Geometry: final body of the model. Coordinates: model frame, mm. A direction names the side the tool comes from. Round coordinates to 2 decimals unless told otherwise and drop trailing zeros. Write each loop counter-clockwise with the first axis right and the second up, starting at its lowest first coordinate (ties: lowest second). Pieces come first, ordered by that corner, then holes. Notation, with made-up numbers: M -5.5,85 L 44.5,85 A11 cw 44.5,105 Z; hole C 24.5,37 d5. An arc over 180 degrees is marked long. Answer as CSV lines item,"result". Start each with the question number.
Q1. Ray query, probe 1 along Y at (x, z) = (8.5, -0.5); probe 2 along Z at (x, y) = (10.25, 9); probe 3 along Y at (x, z) = (6.25, 6.5) (3 decimals). Return the intervals inside material, ascending.
Q2. Reachability of faces 1 (the flat face through (4.13, 9.44, -0.44)), 2 (the flat face through (8.1, 8.152, -0.4)), 3 (the flat face through (8, 9.309, -0.4)) from +Z, -Z, +X, -X, +Y, -Y: full face, straight path, thin tool, end or side. Return the list, or none.
Q3. Section query A-A on z = 7. Output: boundary loops of the cut face in (x, y) (3 decimals), and give its area (3 significant figures).
Q4. Section query B-B on y = 6.1. Output: boundary loops of the cut face in (x, z) (3 decimals), and give its area (3 significant figures).
Q5. First-contact query: pin 1 (1.1 mm diameter, centred on y = 7.5, z = 7.5, fed in from -X); pin 2 (1 mm diameter, centred on x = 2, z = 6, fed in from +Y); pin 3 (0.5 mm diameter, centred on x = 7, z = -0.5, fed in from -Y); pin 4 (1.1 mm diameter, centred on x = 6.5, z = 7, fed in from -Y). Flat tips, straight axial feed; report the tip coordinate or a pass-through.
Q6. Section query C-C on x = 10. Output: boundary loops of the cut face in (y, z), and give its area (3 significant figures).
Q7. Mould query, pull axis X, two halves, no side actions, for faces 4 (the flat face through (5.929, 8.4, -0.4)), 5 (the flat face through (6, 4.075, 7)), 6 (the flat face through (12.14, 6, 2)), 7 (the flat face through (4.9, 6.84, -0.4)). Classes: pulls with the +X half, pulls with the -X half, needs draft (parallel to the pull), parting line crosses it, or undercut.
Autodesk Inventor part; units mm, degrees
ref_plane "Work Plane1" through (0, 0, 5) normal (0, 0, 1) x (1, 0, 0)
ref_plane "YZ Plane" through (0, 0, 0) normal (1, 0, 0) x (0, 1, 0)
ref_plane "XZ Plane" through (0, 0, 0) normal (0, 1, 0) x (-1, 0, 0)
sketch "Sketch1" plane through (0, 0, 0) normal (0, 0, 1) x (1, 0, 0)
  line L0 (14.6962, 12.74) -> (14.6962, 0) construction
  line L1 (10.61, 12.2) -> (1.53, 12.2)
  arc A0 (1.53, 12.2) -> (0, 10.67) centre (1.53, 10.67) ccw
  line L2 (0, 10.67) -> (0, 1.53)
  arc A1 (0, 1.53) -> (1.53, 0) centre (1.53, 1.53) ccw
  line L3 (1.53, 0) -> (10.61, 0)
  arc A2 (10.61, 0) -> (12.14, 1.53) centre (10.61, 1.53) ccw
  arc A3 (12.14, 10.67) -> (10.61, 12.2) centre (10.61, 10.67) ccw
  line L4 (12.14, 10.67) -> (12.14, 1.53)
  point P0 (0, 0)
  point P1 (0, 0)
  dimension "d10" = 12.74
ref_plane "Work Plane1" through (0, 0, 5) normal (0, 0, 1) x (1, 0, 0)
sketch "Sketch2" plane through (0, 0, 5) normal (0, 0, 1) x (1, 0, 0)
  line L0 (10.88, 12.74) -> (1.8, 12.74)
  line L1 (10.88, 12.74) -> (1.8, 12.74)
  arc A0 (1.8, 12.74) -> (0, 10.94) centre (1.8, 10.94) ccw
  line L2 (0, 10.94) -> (0, 1.8)
  arc A1 (0, 1.8) -> (1.8, 0) centre (1.8, 1.8) ccw
  line L3 (1.8, 0) -> (10.88, 0)
  arc A2 (10.88, 0) -> (12.68, 1.8) centre (10.88, 1.8) ccw
  line L4 (12.68, 1.8) -> (12.68, 10.94)
  arc A3 (12.68, 10.94) -> (10.88, 12.74) centre (10.88, 10.94) ccw
  circle A4 centre (6.34, 6.37) radius 2.8
  line L5 (5.665, 8.395) -> (7.015, 8.395)
  line L6 (7.015, 4.345) -> (5.665, 4.345)
  line L7 (5.665, 4.345) -> (7.015, 8.395) construction
  line L8 (5.665, 8.395) -> (7.015, 4.345) construction
  line L9 (8.365, 5.695) -> (8.365, 7.045)
  line L10 (4.315, 7.045) -> (4.315, 5.695)
  line L11 (4.315, 5.695) -> (8.365, 7.045) construction
  line L12 (8.365, 5.695) -> (4.315, 7.045) construction
  line L13 (4.315, 5.695) -> (5.665, 5.695)
  line L14 (7.015, 5.695) -> (8.365, 5.695)
  line L15 (5.665, 4.345) -> (5.665, 5.695)
  line L16 (5.665, 7.045) -> (5.665, 8.395)
  line L17 (8.365, 7.045) -> (7.015, 7.045)
  line L18 (5.665, 7.045) -> (4.315, 7.045)
  line L19 (7.015, 8.395) -> (7.015, 7.045)
  line L20 (7.015, 5.695) -> (7.015, 4.345)
  point P0 (0, 0)
  dimension "d3" = 5.6
  dimension "d4" = 4.05
  dimension "d5" = 1.35
  dimension "d6" = 4.05
  dimension "d7" = 1.35
extrude "Extrusion3" add sketch "Sketch1" along normal blind 5
sketch "Sketch3" plane through (0, 0, 5) normal (0, 0, 1) x (1, 0, 0)
  line L0 (10.61, 12.47) -> (1.53, 12.47)
  line L1 (10.61, 12.47) -> (1.53, 12.47)
  arc A0 (1.53, 12.47) -> (-0.27, 10.67) centre (1.53, 10.67) ccw
  line L2 (-0.27, 10.67) -> (-0.27, 1.53)
  arc A1 (-0.27, 1.53) -> (1.53, -0.27) centre (1.53, 1.53) ccw
  line L3 (1.53, -0.27) -> (10.61, -0.27)
  arc A2 (10.61, -0.27) -> (12.41, 1.53) centre (10.61, 1.53) ccw
  line L4 (12.41, 1.53) -> (12.41, 10.67)
  arc A3 (12.41, 10.67) -> (10.61, 12.47) centre (10.61, 10.67) ccw
  circle A4 centre (6.07, 6.1) radius 2.8
  line L5 (5.395, 8.125) -> (6.745, 8.125)
  line L6 (6.745, 4.075) -> (5.395, 4.075)
  line L7 (5.395, 4.075) -> (6.745, 8.125) construction
  line L8 (5.395, 8.125) -> (6.745, 4.075) construction
  line L9 (8.095, 5.425) -> (8.095, 6.775)
  line L10 (4.045, 6.775) -> (4.045, 5.425)
  line L11 (4.045, 5.425) -> (8.095, 6.775) construction
  line L12 (8.095, 5.425) -> (4.045, 6.775) construction
  line L13 (4.045, 5.425) -> (5.395, 5.425)
  line L14 (6.745, 5.425) -> (8.095, 5.425)
  line L15 (5.395, 4.075) -> (5.395, 5.425)
  line L16 (5.395, 6.775) -> (5.395, 8.125)
  line L17 (8.095, 6.775) -> (6.745, 6.775)
  line L18 (5.395, 6.775) -> (4.045, 6.775)
  line L19 (6.745, 8.125) -> (6.745, 6.775)
  line L20 (6.745, 5.425) -> (6.745, 4.075)
  line L21 (10.61, 12.2) -> (1.53, 12.2)
  line L22 (0, 10.67) -> (0, 1.53)
  point P0 (0, 0)
  point P1 (-0.27, -0.27)
  point P2 (6.07, 12.2)
  point P3 (0, 6.1)
  point P4 (6.07, 6.1)
  dimension "d14" = 5.6
  dimension "d15" = 4.05
  dimension "d16" = 1.35
  dimension "d17" = 4.05
  dimension "d18" = 1.35
extrude "Extrusion4" add sketch "Sketch3" along normal blind 4.8 contours A4
sketch "Sketch4" plane through (0, 0, 0) normal (0, 0, -1) x (-1, 0, 0)
  line L0 (-13.9436, 0) -> (-13.9436, 2.266)
  line L1 (-15.5559, 0) -> (-15.5559, 6.84)
  line L2 (-1.53, 0) -> (-10.61, 0)
  line L3 (-9.7626, 9.89) -> (-2.3774, 9.89) construction
  line L4 (-2.3774, 9.89) -> (-2.3774, 6.84) construction
  line L5 (-2.3774, 6.84) -> (-9.7626, 6.84) construction
  line L6 (-9.7626, 6.84) -> (-9.7626, 9.89) construction
  line L7 (-7.4059, 5.4569) -> (-4.7341, 5.4569) construction
  line L8 (-4.7341, 5.4569) -> (-4.7341, 2.266) construction
  line L9 (-4.7341, 2.266) -> (-7.4059, 2.266) construction
  line L10 (-7.4059, 2.266) -> (-7.4059, 5.4569) construction
  line L11 (-7.4047, 9.3092) -> (-8.685, 9.3092)
  line L12 (-8.685, 9.3092) -> (-8.685, 8.7333)
  line L13 (-8.685, 8.7333) -> (-7.506, 8.7333)
  line L14 (-7.506, 8.7333) -> (-7.506, 8.1524)
  line L15 (-7.506, 8.1524) -> (-8.685, 8.1524)
  line L16 (-8.685, 8.1524) -> (-8.685, 6.84)
  line L17 (-8.685, 6.84) -> (-9.4463, 6.84)
  line L18 (-9.4463, 6.84) -> (-9.4463, 9.89)
  line L19 (-9.4463, 9.89) -> (-7.4047, 9.89)
  line L20 (-7.4047, 9.89) -> (-7.4047, 9.3092)
  line L21 (-5.4916, 6.84) -> (-7.1328, 6.84)
  line L22 (-7.1328, 6.84) -> (-7.1328, 7.3714)
  line L23 (-7.1328, 7.3714) -> (-6.6953, 7.3714)
  line L24 (-6.6953, 7.3714) -> (-6.6953, 9.3586)
  line L25 (-6.6953, 9.3586) -> (-7.1328, 9.3586)
  line L26 (-7.1328, 9.3586) -> (-7.1328, 9.89)
  line L27 (-7.1328, 9.89) -> (-5.4916, 9.89)
  line L28 (-5.4916, 9.89) -> (-5.4916, 9.3586)
  line L29 (-5.4916, 9.3586) -> (-5.9291, 9.3586)
  line L30 (-5.9291, 9.3586) -> (-5.9291, 7.3714)
  line L31 (-5.9291, 7.3714) -> (-5.4916, 7.3714)
  line L32 (-5.4916, 7.3714) -> (-5.4916, 6.84)
  line L33 (-2.4021, 6.84) -> (-3.2869, 6.84)
  line L34 (-3.2869, 6.84) -> (-3.8752, 7.8114)
  line L35 (-3.8752, 7.8114) -> (-4.4758, 6.84)
  line L36 (-4.4758, 6.84) -> (-5.3236, 6.84)
  line L37 (-5.3236, 6.84) -> (-4.3324, 8.3749)
  line L38 (-4.3324, 8.3749) -> (-5.284, 9.89)
  line L39 (-5.284, 9.89) -> (-4.3992, 9.89)
  line L40 (-4.3992, 9.89) -> (-3.848, 8.9681)
  line L41 (-3.848, 8.9681) -> (-3.282, 9.89)
  line L42 (-3.282, 9.89) -> (-2.4342, 9.89)
  line L43 (-2.4342, 9.89) -> (-3.3907, 8.407)
  line L44 (-3.3907, 8.407) -> (-2.4021, 6.84)
  spline S0 degree 2 poles (-4.8626, 3.1854) (-4.8626, 2.9902) (-5.0257, 2.6516) (-5.1814, 2.528) knots 0 0 0 1 2 2 2
  spline S1 degree 2 poles (-5.1814, 2.528) (-5.3372, 2.4044) (-5.7845, 2.266) (-6.0737, 2.266) knots 0 0 0 1 2 2 2
  spline S2 degree 2 poles (-6.0737, 2.266) (-6.3827, 2.266) (-6.8449, 2.4069) (-6.9932, 2.528) knots 0 0 0 1 2 2 2
  spline S3 degree 2 poles (-6.9932, 2.528) (-7.139, 2.6491) (-7.2774, 2.9778) (-7.2774, 3.1607) knots 0 0 0 1 2 2 2
  spline S4 degree 2 poles (-7.2774, 3.1607) (-7.2774, 3.4227) (-6.9882, 3.7712) (-6.7139, 3.8874) knots 0 0 0 1 2 2 2
  line L45 (-6.7139, 3.8874) -> (-6.7139, 3.8998)
  spline S5 degree 2 poles (-6.7139, 3.8998) (-6.9833, 4.0307) (-7.1958, 4.404) (-7.1958, 4.6338) knots 0 0 0 1 2 2 2
  spline S6 degree 2 poles (-7.1958, 4.6338) (-7.1958, 4.8019) (-7.0475, 5.096) (-6.9017, 5.2122) knots 0 0 0 1 2 2 2
  spline S7 degree 2 poles (-6.9017, 5.2122) (-6.7608, 5.3234) (-6.3332, 5.4569) (-6.0663, 5.4569) knots 0 0 0 1 2 2 2
  spline S8 degree 2 poles (-6.0663, 5.4569) (-5.7845, 5.4569) (-5.3643, 5.3358) (-5.2284, 5.2369) knots 0 0 0 1 2 2 2
  spline S9 degree 2 poles (-5.2284, 5.2369) (-5.09, 5.138) (-4.9417, 4.8513) (-4.9417, 4.6857) knots 0 0 0 1 2 2 2
  spline S10 degree 2 poles (-4.9417, 4.6857) (-4.9417, 4.4682) (-5.1938, 4.1197) (-5.4533, 3.9986) knots 0 0 0 1 2 2 2
  line L46 (-5.4533, 3.9986) -> (-5.4533, 3.9887)
  spline S11 degree 2 poles (-5.4533, 3.9887) (-5.1493, 3.8651) (-4.8626, 3.4647) (-4.8626, 3.1854) knots 0 0 0 1 2 2 2
  spline S12 degree 2 poles (-5.6189, 3.1533) (-5.6189, 3.3041) (-5.7475, 3.4623) (-5.9551, 3.5636) knots 0 0 0 1 2 2 2
  spline S13 degree 2 poles (-5.9551, 3.5636) (-6.0144, 3.5908) (-6.2393, 3.6773) (-6.3258, 3.7144) knots 0 0 0 1 2 2 2
  spline S14 degree 2 poles (-6.3258, 3.7144) (-6.4049, 3.6353) (-6.531, 3.398) (-6.531, 3.2571) knots 0 0 0 1 2 2 2
  spline S15 degree 2 poles (-6.531, 3.2571) (-6.531, 3.0446) (-6.2591, 2.79) (-6.0391, 2.79) knots 0 0 0 1 2 2 2
  spline S16 degree 2 poles (-6.0391, 2.79) (-5.9773, 2.79) (-5.8241, 2.8295) (-5.7648, 2.8691) knots 0 0 0 1 2 2 2
  spline S17 degree 2 poles (-5.7648, 2.8691) (-5.698, 2.916) (-5.6189, 3.0446) (-5.6189, 3.1533) knots 0 0 0 1 2 2 2
  spline S18 degree 2 poles (-5.6857, 4.5968) (-5.6857, 4.7525) (-5.8908, 4.9378) (-6.0663, 4.9378) knots 0 0 0 1 2 2 2
  spline S19 degree 2 poles (-6.0663, 4.9378) (-6.2344, 4.9378) (-6.4395, 4.7698) (-6.4395, 4.6462) knots 0 0 0 1 2 2 2
  spline S20 degree 2 poles (-6.4395, 4.6462) (-6.4395, 4.5251) (-6.3159, 4.3743) (-6.1849, 4.3125) knots 0 0 0 1 2 2 2
  spline S21 degree 2 poles (-6.1849, 4.3125) (-6.1281, 4.2829) (-5.9699, 4.2211) (-5.8389, 4.1716) knots 0 0 0 1 2 2 2
  spline S22 degree 2 poles (-5.8389, 4.1716) (-5.7598, 4.2754) (-5.6857, 4.4707) (-5.6857, 4.5968) knots 0 0 0 1 2 2 2
  point P0 (0, 0)
  point P1 (-6.07, 0)
  point P2 (-6.07, 2.266)
  point P3 (-6.07, 6.84)
  point P4 (-6.07, 6.84)
  point P5 (-6.07, 2.266)
  dimension "d21" = 2.266
  dimension "d22" = 6.84
extrude "Extrusion5" add sketch "Sketch4" along normal blind 0.9
properties part number "IPC FIX 8"
Entries:
1,probe 1,"y = 8.15 to 8.73, 9.31 to 9.89"
1,probe 2,"z = 0 to 5"
1,probe 3,"y = 3.306 to 4.075, 8.125 to 8.894"
2,face 1,"-Z, +Y"
2,face 2,"-Z, -Y"
2,face 3,"-Z"
3,outline,"C 6.07,6.1 d5.6; hole M 4.045,5.425 L 5.395,5.425 L 5.395,4.075 L 6.745,4.075 L 6.745,5.425 L 8.095,5.425 L 8.095,6.775 L 6.745,6.775 L 6.745,8.125 L 5.395,8.125 L 5.395,6.775 L 4.045,6.775 Z"
3,area,"15.5 mm^2"
4,outline,"M 0,0 L 12.14,0 L 12.14,5 L 8.87,5 L 8.87,9.8 L 8.095,9.8 L 8.095,5 L 4.045,5 L 4.045,9.8 L 3.27,9.8 L 3.27,5 L 0,5 Z"
4,area,"68.1 mm^2"
5,pin 1,"stops at x = 3.4"
5,pin 2,"passes through"
5,pin 3,"stops at y = 2.39"
5,pin 4,"stops at y = 3.3"
6,outline,"M 0,0 L 12.2,0 L 12.2,5 L 0,5 Z"
6,area,"61.0 mm^2"
7,face 4,"undercut"
7,face 5,"undercut"
7,face 6,"pulls with the +X half"
7,face 7,"needs draft"
